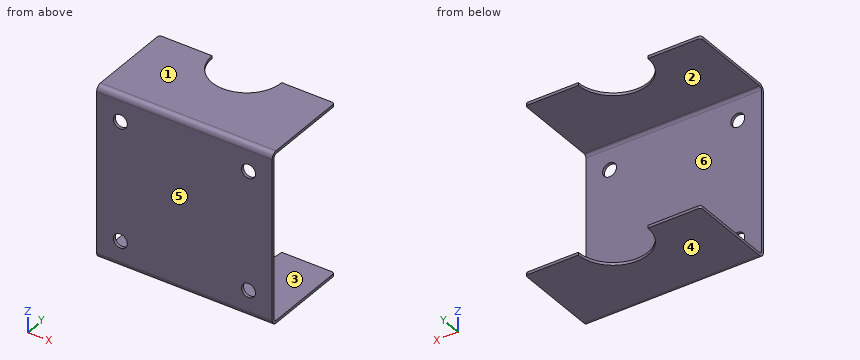
Autodesk Inventor part; units mm, degrees
ref_plane "YZ Plane" through (0, 0, 0) normal (1, 0, 0) x (0, 1, 0)
ref_plane "XZ Plane" through (0, 0, 0) normal (0, 1, 0) x (-1, 0, 0)
ref_plane "XY Plane" through (0, 0, 0) normal (0, 0, 1) x (1, 0, 0)
sketch "Sketch4" plane through (0, 0, 0) normal (0, 1, 0) x (-1, 0, 0)
  line L0 (63, -57.5) -> (-63, -57.5)
  line L1 (-63, -57.5) -> (-63, 57.5)
  line L2 (-63, 57.5) -> (63, 57.5)
  line L3 (63, 57.5) -> (63, -57.5)
  line L4 (63, -57.5) -> (-63, 57.5) construction
  point P0 (0, 0)
  point P1 (0, 0)
  dimension "d24" = 126
  dimension "d25" = 115
extrude "Plate4" add sketch "Sketch4" along normal mid plane 2
sketch "Sketch5" plane through (63, 3, 59.5) normal (0, 0, 1) x (1, 0, 0)
  line L0 (-126, 0) -> (0, 0)
  line L1 (0, 0) -> (0, 61)
  line L2 (0, 61) -> (-126, 61)
  line L3 (-126, 61) -> (-126, 0)
edge flange "Flange3" height 65 angle 90 thickness 2 bend radius 2 thickness toward (0, 0, 1) relief tear relief width 2 relief depth 1 corner gap 2 corner form 0 edges at (0, 1, 57.5) (0, 1, -57.5) wall of the first edge with corners at (-63, 3, 59.5) (63, 3, 59.5) (63, 64, 59.5) (-63, 64, 59.5)
bend "Bend3"
corner "Corner3"
sketch "Sketch6" plane through (-63, 64, 61.5) normal (0, 0, 1) x (1, 0, 0)
  line L0 (0, 0) -> (126, 0)
  circle A0 centre (63, 0) radius 25
  point P0 (63, -64)
  dimension "d37" = 50
extrude "Extrusion1" cut sketch "Sketch6" against normal through all
fillet "Fillet1" radius 2 4 edges at (-63, 64, -60.5) (63, 64, -60.5) (63, 64, 60.5) (-63, 64, 60.5)
sketch "Sketch7" plane through (0, -1, 0) normal (0, -1, 0) x (1, 0, 0)
  circle A0 centre (46, -42.5) radius 5
  line L0 (63, 57.5) -> (63, -57.5)
  line L1 (63, -57.5) -> (-63, -57.5)
  line L2 (25, 59.5) -> (-25, 59.5) construction
  line L3 (0, -74.3103) -> (0, 74.3103) construction
  line L4 (114.9724, 0) -> (-114.9724, 0) construction
  circle A1 centre (-46, -42.5) radius 5
  circle A2 centre (46, 42.5) radius 5
  circle A3 centre (-46, 42.5) radius 5
  point P0 (0, 0)
  point P1 (0, 0)
  dimension "d41" = 10
  dimension "d42" = 17
  dimension "d43" = 15
extrude "Extrusion2" cut sketch "Sketch7" against normal up to surface (2 mm away)
equation "\"d26\" = Thickness"
equation "\"d27\" = BendReliefWidth"
equation "\"d28\" = BendReliefDepth"
equation "\"d29\" = MinimumRemnant"
equation "\"d30\" = TransitionRadius"
equation "\"d33\" = BendRadius"
equation "\"d34\" = CornerReliefSize"
equation "\"d35\" = GapSize"
equation "\"d36\" = JacobiRadiusSize"
equation "\"BendRadius\" = Thickness"
equation "\"BendReliefWidth\" = Thickness"
equation "\"BendReliefDepth\" = 0.5 * Thickness"
equation "\"CornerReliefSize\" = 4 * Thickness"
equation "\"MinimumRemnant\" = 2 * Thickness"
equation "\"TransitionRadius\" = BendRadius"
equation "\"JacobiRadiusSize\" = BendRadius"
equation "\"GapSize\" = Thickness"
properties part number "Крепление"
The model under review builds one solid part; all positions refer to its coordinate system, in mm. Face numbers are marked on the shaded views. A direction names the side the tool comes from. Round coordinates to 2 decimals unless told otherwise and drop trailing zeros. Order: outer loops, then holes, each group sorted by start corner. A loop starts at its lowest first (then second) coordinate and runs counter-clockwise, first axis right, second up. Notation, with made-up numbers: (43, 32.25) - (72, 32.25) arc R15 ccw to (72, 36.25) - close; hole circle Ø3 at (20, 38). An arc over 180 degrees is marked (long way). Answer in a Markdown table with one row per item.
(1) Mouldability with a two-part tool opening along Z and no side actions: class the marked faces 1, 2, 3 and 4 as released by +Z, released by -Z, zero draft, split by the parting line, or undercut.
Result set:
| item | result |
|---|---|
| face 1 | released by +Z |
| face 2 | undercut |
| face 3 | undercut |
| face 4 | released by -Z |
(2) For line 1 (Z direction, x = 1.5, y = 26.5); line 2 (Z direction, x = -46, y = 0.4); line 3 (Z direction, x = 46, y = -0.55), list the stretches that pass through material, from the lowest coordinate up. Write a range as from..to.
Result set:
| item | result |
|---|---|
| line 1 | z = -61.5..-59.5, 59.5..61.5 |
| line 2 | z = -60.54..-47.5, -37.5..37.5, 47.5..60.54 |
| line 3 | z = -59.34..-47.5, -37.5..37.5, 47.5..59.34 |
(3) Take a section at D-D on x = 33.5. Write out the cut boundary in (y, z), plus the area to 3 significant figures.
Result set:
| item | result |
|---|---|
| outline | (-1, -57.5) arc R4 ccw to (3, -61.5) - (64, -61.5) - (64, -59.5) - (3, -59.5) arc R2 cw to (1, -57.5) - (1, 57.5) arc R2 cw to (3, 59.5) - (64, 59.5) - (64, 61.5) - (3, 61.5) arc R4 ccw to (-1, 57.5) - close |
| area | 493 mm2 |
(4) Take a section at A-A on x = -46. Write out the cut boundary in (y, z), plus the area to 3 significant figures.
Result set:
| item | result |
|---|---|
| outline | (-1, -57.5) arc R4 ccw to (3, -61.5) - (64, -61.5) - (64, -59.5) - (3, -59.5) arc R2 cw to (1, -57.5) - (1, -47.5) - (-1, -47.5) - close; (-1, -37.5) - (1, -37.5) - (1, 37.5) - (-1, 37.5) - close; (-1, 47.5) - (1, 47.5) - (1, 57.5) arc R2 cw to (3, 59.5) - (64, 59.5) - (64, 61.5) - (3, 61.5) arc R4 ccw to (-1, 57.5) - close |
| area | 453 mm2 |
(5) Machinability: for the marked faces 5 and 6, which of the approach directions +Z, -Z, +X, -X, +Y, -Y give a long, thin tool a straight path to every point of the face, cutting with its end or side? Answer none if there is none.
Result set:
| item | result |
|---|---|
| face 5 | +Z, -Z, +X, -X, -Y |
| face 6 | +X, -X, +Y |
(6) Clearance check with flat-ended pins moving along their axes: P1, Ø8, axis at x = 46, z = -42.5, coming from the +Y side; P2, Ø2, axis at x = -2, z = -26.5, coming from the +Y side. State where each tip first meets the part, or that it passes through.
Result set:
| item | result |
|---|---|
| P1 | passes through |
| P2 | stops at y = 1 |
(7) Take a section at B-B on z = 42.5. Write out the cut boundary in (x, y).
Result set:
| item | result |
|---|---|
| outline | (-63, -1) - (-51, -1) - (-51, 1) - (-63, 1) - close; (-41, -1) - (41, -1) - (41, 1) - (-41, 1) - close; (51, -1) - (63, -1) - (63, 1) - (51, 1) - close |
(8) Take a section at C-C on y = 33.5. Write out the cut boundary in (x, z).
Result set:
| item | result |
|---|---|
| outline | (-63, -61.5) - (63, -61.5) - (63, -59.5) - (-63, -59.5) - close; (-63, 59.5) - (63, 59.5) - (63, 61.5) - (-63, 61.5) - close |
